Check sheet for the modelled part. Datum: model origin and axes. Units: mm. A direction names the side the tool comes from. Coordinates: 2 decimals unless noted, no trailing zeros. Loops run counter-clockwise (first coordinate to the right, second up) from the corner with the lowest first, then second, coordinate; pieces in that order, holes last. Notation, with made-up numbers: (-28.5, 88.25) - (-20.5, 88.25) arc R24 ccw to (-20.5, 118.25) - close; hole circle Ø9 at (88, 33). An arc over 180 degrees is marked (long way). Write each question's results on one line, items separated by ' | '. Start each with the question number.
1. Cross-section at D-D (y = 667). Record the cut outline in (x, z), and give its area (3 significant figures).
2. Tool access check on faces 5 (the face through (439.645, 406, -488)), 6 (the face through (0.66, 394.4, -39.985)), 7 (the face through (229, 812, -475)), 8 (the face through (-464.645, 394, -488)). Record the directions out of +Z, -Z, +X, -X, +Y, -Y that give a thin tool (end or side, any length) a straight path to the whole face; none if there is none.
3. Gauge pin test, flat ends, axial feed: P1, Ø17.5, axis at x = 0, z = -25, coming from the +Y side; P2, Ø12.5, axis at y = 206.5, z = -492.5, coming from the +X side; P3, Ø12.5, axis at y = 809.5, z = -229.5, coming from the +X side. Record the tip position at first contact, or that the pin passes through.
4. Cross-section at B-B (z = -326). Record the cut outline in (x, y).
5. Thickness scan on line 1 (Y direction, x = -326, z = -352.5); line 2 (Z direction, x = 0, y = 821.25); line 3 (X direction, y = 363, z = -25). Record the ranges inside material, lowest first. Write a range as [from, to].
6. Cross-section at A-A (y = 315). Record the cut outline in (x, z), and give its area (3 significant figures).
7. Cross-section at C-C (x = 299.5). Record the cut outline in (y, z), and give its area (3 significant figures).
8. Draft check along X on faces 1 (the face through (2, 398, -500)), 2 (the face through (-247, -12, -247)), 3 (the face through (-1.888, -21.549, -10.623)), 4 (the face through (-12.5, 812, -258)). Enter one of: released by +X, released by -X, zero draft, split by the parting line, or undercut.
```python
from build123d import *

# Parameters (mm, degrees)
F1_DEPTH       = 25
F6_D           = 17
F6_DEPTH       = 100
F6_CBORE_D     = 29
F6_CBORE_DEPTH = 7
F6_TIP         = 5.1073152617
F8_D           = 17
F8_DEPTH       = 100
F8_CBORE_D     = 29
F8_CBORE_DEPTH = 7
F8_TIP         = 5.1073152617
F9_DEPTH       = 400
F12_DEPTH      = 25
F13_W          = 25
F13_H          = 25
F14_DEPTH      = 800
F15_W          = 25
F15_H          = 25
F16_DEPTH      = 800


with BuildPart() as f1:
    # F0 (on Front) → F1 (new body)
    with BuildSketch(Plane.XZ):
        Polygon((-500, -500), (0, -500), (500, -500), (0, 0), align=None)
        Polygon((-12.5, -47.8553390593), (-12.5, -475), (-439.6446609407, -475), align=None, mode=Mode.SUBTRACT)
        Polygon((439.6446609407, -475), (12.5, -475), (12.5, -47.8553390593), align=None, mode=Mode.SUBTRACT)
    extrude(amount=F1_DEPTH)


with BuildPart() as f3_1:
    # F3: instance of F1
    add(f1.part.mirror(Plane.XZ.offset(-400)))

    # F6
    with Locations(Plane(origin=(0, 825, 0), x_dir=(-1, 0, 0), z_dir=(0, 1, 0))):
        with Locations((0, -25)):
            CounterBoreHole(F6_D / 2, F6_CBORE_D / 2, F6_CBORE_DEPTH, depth=F6_DEPTH)
            with Locations((0, 0, -(F6_DEPTH + F6_TIP / 2))):  # 118° drill point
                Cone(0, F6_D / 2, F6_TIP, mode=Mode.SUBTRACT)


with BuildPart() as f1_1:
    add(f1.part)

    # F8
    with Locations(Plane.XZ.offset(25)):
        with Locations((0, -25)):
            CounterBoreHole(F8_D / 2, F8_CBORE_D / 2, F8_CBORE_DEPTH, depth=F8_DEPTH)
            with Locations((0, 0, -(F8_DEPTH + F8_TIP / 2))):  # 118° drill point
                Cone(0, F8_D / 2, F8_TIP, mode=Mode.SUBTRACT)

    # F4 (on face) → F9 (join)
    with BuildSketch(Plane(origin=(0, 0, 0), x_dir=(-1, 0, 0), z_dir=(0, 1, 0))):
        with BuildLine():
            ThreePointArc((15, -25), (10.6066017178, -14.3933982822), (0, -10))
            ThreePointArc((0, -10), (-10.6066017178, -35.6066017178), (15, -25))
        make_face()
        with BuildLine():
            ThreePointArc((8.5, -25), (-6.0104076401, -31.0104076401), (0, -16.5))
            ThreePointArc((0, -16.5), (6.0104076401, -18.9895923599), (8.5, -25))
        make_face(mode=Mode.SUBTRACT)
    extrude(amount=F9_DEPTH)



with BuildPart() as f1_2:
    add(f1_1.part)

    add(f3_1.part)  # F10 merges F3_1
    # F10: F1 across plane
    add(f1_1.part.mirror(Plane.XZ.offset(-400)))

    # F11 (on face) → F12 (join)
    with BuildSketch(Plane.XY.offset(-475)):
        Polygon((12.4637438569, 800), (-12.5, 800), (-12.5, 0), (12.9191244142, 0), align=None)
    extrude(amount=-F12_DEPTH)

    # F13 (on face) → F14 (join)
    with BuildSketch(Plane.XZ.offset(-800)):
        with Locations((452.1446609407, -487.5)):
            Rectangle(F13_W, F13_H)
    extrude(amount=F14_DEPTH)

    # F15 (on face) → F16 (join)
    with BuildSketch(Plane(origin=(0, 0, 0), x_dir=(-1, 0, 0), z_dir=(0, 1, 0))):
        with Locations((452.1446609407, -487.5)):
            Rectangle(F15_W, F15_H)
    extrude(amount=F16_DEPTH)


solid = f1_2.part
```
Established:
1) outline: (-464.64, -500) - (-439.64, -500) - (-439.64, -475) - (-464.64, -475) - close; circle Ø30 at (0, -25); (-12.5, -500) - (12.54, -500) - (12.54, -475) - (-12.5, -475) - close; (439.64, -500) - (464.64, -500) - (464.64, -475) - (439.64, -475) - close; hole circle Ø17 at (0, -25) | area: 2,360 mm^2
2) face 5: +Z, -Z | face 6: none | face 7: +Y, -Y | face 8: +Z, -Z, -X
3) P1: y = 818 | P2: x = 464.64 | P3: x = 235.75
4) outline: (-326, -25) - (-290.64, -25) - (-290.64, 0) - (-326, 0) - close; (-326, 800) - (-290.64, 800) - (-290.64, 825) - (-326, 825) - close; (-12.5, -25) - (12.5, -25) - (12.5, 0) - (-12.5, 0) - close; (-12.5, 800) - (12.5, 800) - (12.5, 825) - (-12.5, 825) - close; (290.64, -25) - (326, -25) - (326, 0) - (290.64, 0) - close; (290.64, 800) - (326, 800) - (326, 825) - (290.64, 825) - close
5) line 1: [-25, 0], [800, 825] | line 2: [-500, -39.5], [-10.5, 0] | line 3: [-15, -8.5], [8.5, 15]
6) outline: (-464.64, -500) - (-439.64, -500) - (-439.64, -475) - (-464.64, -475) - close; circle Ø30 at (0, -25); (-12.5, -500) - (12.74, -500) - (12.74, -475) - (-12.5, -475) - close; (439.64, -500) - (464.64, -500) - (464.64, -475) - (439.64, -475) - close; hole circle Ø17 at (0, -25) | area: 2,360 mm^2
7) outline: (-25, -500) - (0, -500) - (0, -475) - (-25, -475) - close; (-25, -334.86) - (0, -334.86) - (0, -299.5) - (-25, -299.5) - close; (800, -500) - (825, -500) - (825, -475) - (800, -475) - close; (800, -334.86) - (825, -334.86) - (825, -299.5) - (800, -299.5) - close | area: 3,020 mm^2
8) face 1: zero draft | face 2: released by -X | face 3: undercut | face 4: undercut
